Could you check a few things on this model? Use its own coordinates, in mm. Face numbers are marked on the shaded views. A direction names the side the tool comes from. Give positions to 0.01 mm unless a question says otherwise; leave off trailing zeros. Loops run counter-clockwise (first coordinate to the right, second up) from the corner with the lowest first, then second, coordinate; pieces in that order, holes last. Notation, with made-up numbers: (-35.75, 62.5) - (21.25, 62.5) arc R32 cw to (21.25, 101.5) - close; hole circle Ø10 at (10, 23). An arc over 180 degrees is marked (long way). Write each question's results on one line, items separated by ' | '. Start each with the question number.
(1) Suppose I cut it at D-D (y = -15.5). Please give me the cut outline in (x, z), and give its area (3 significant figures).
(2) Suppose I cut it at A-A (z = 19.5). Please give me the cut outline in (x, y), and give its area (3 significant figures).
(3) Suppose I cut it at C-C (x = 42). Please give me the cut outline in (y, z).
(4) On a 3-axis mill with a long thin cutter (end or side, diameter ignored), from which of +Z, -Z, +X, -X, +Y, -Y can I reach the whole of each face in a straight line? I mean the marked faces 5 and 6. Say none if no direction works.
(5) Suppose I cut it at B-B (y = 41). Please give me the cut outline in (x, z), and give its area (3 significant figures).
(6) I need wall thicknesses on line 1 (Y direction, x = 35.5, z = 36.5); line 2 (Y direction, x = 24, z = 5). Which ranges of each line are inside material? Lowest first, please.
(7) For pin 1 (13.5 mm diameter, centred on x = -19.5, y = -18, fed in from +Z), with a flat end and sliding along its axis, tell me the tip position at first contact or that it passes through.
(8) If we mould it in two halves opening along Y, with no side actions, what happens to the marked faces 1, 2, 3 and 4? For each: released by +Y, released by -Y, zero draft, split by the parting line, or undercut.
from build123d import *

# Parameters (mm, degrees)
F0_W     = 101.6
F0_H     = 101.6
F0_W_2   = 91.44
F0_H_2   = 91.44
F2_DEPTH = 101.6
F1_W     = 91.44
F1_H     = 45.72
F3_DEPTH = 5.08


with BuildPart() as f2:
    # F0 (on Top) → F2 (new body)
    with BuildSketch(Plane.XY):
        Rectangle(F0_W, F0_H)
        Rectangle(F0_W_2, F0_H_2, mode=Mode.SUBTRACT)
    extrude(amount=F2_DEPTH)

    # F1 (on face) → F3 (join)
    with BuildSketch(Plane.XY):
        with Locations((0, -22.86)):
            Rectangle(F1_W, F1_H)
    extrude(amount=F3_DEPTH)


solid = f2.part
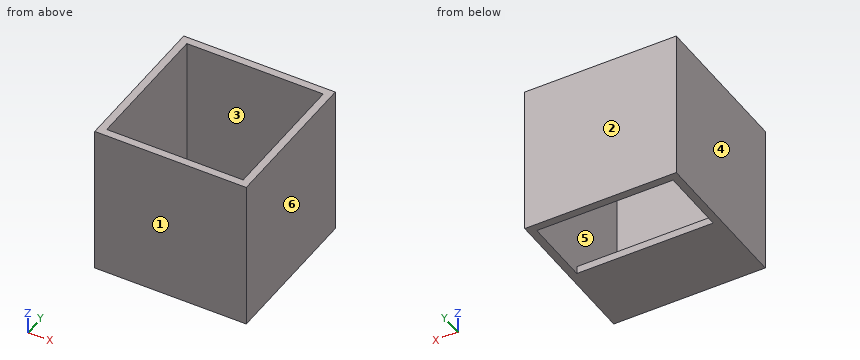
Output values:
1) outline: (-50.8, 0) - (50.8, 0) - (50.8, 101.6) - (45.72, 101.6) - (45.72, 5.08) - (-45.72, 5.08) - (-45.72, 101.6) - (-50.8, 101.6) - close | area: 1,500 mm2
2) outline: (-50.8, -50.8) - (50.8, -50.8) - (50.8, 50.8) - (-50.8, 50.8) - close; hole (-45.72, -45.72) - (45.72, -45.72) - (45.72, 45.72) - (-45.72, 45.72) - close | area: 1,960 mm2
3) outline: (-50.8, 0) - (0, 0) - (0, 5.08) - (-45.72, 5.08) - (-45.72, 101.6) - (-50.8, 101.6) - close; (45.72, 0) - (50.8, 0) - (50.8, 101.6) - (45.72, 101.6) - close
4) face 5: +Z | face 6: +Z, -Z, +X, +Y, -Y
5) outline: (-50.8, 0) - (-45.72, 0) - (-45.72, 101.6) - (-50.8, 101.6) - close; (45.72, 0) - (50.8, 0) - (50.8, 101.6) - (45.72, 101.6) - close | area: 1,030 mm2
6) line 1: -50.8 to -45.72, 45.72 to 50.8 | line 2: -50.8 to 0, 45.72 to 50.8
7) pin 1: z = 5.08
8) face 1: released by -Y | face 2: released by +Y | face 3: undercut | face 4: zero draft
